Geometry: final body of the model. Coordinates: model frame, mm. A direction names the side the tool comes from. Give positions to 0.01 mm unless a question says otherwise; leave off trailing zeros. Loops run counter-clockwise (first coordinate to the right, second up) from the corner with the lowest first, then second, coordinate; pieces in that order, holes last. Notation, with made-up numbers: (-23.75, -22) -> (-18.75, -22) arc R13 ccw to (-18.75, 1) -> close; hole circle Ø2 at (-31.5, 45). An arc over 180 degrees is marked (long way). Answer in a Markdown table with one row per item. Add a question column.
1) Draft query along X for faces 1 (the flat face through (43, 43.18, -1)), 2 (the flat face through (4, 10.16, -60)), 3 (the flat face through (0, 21, -31)). Return one class per face: +X half, -X half, draft (parallel to the pull), parting line (faces both ways), or undercut.
2) Section query D-D (x = 5.08). Return the cut outline in (y, z).
3) Access query for faces 4 (the flat face through (60, 21, 0)), 5 (the flat face through (7.62, 8, -58)). Directions: +Z, -Z, +X, -X, +Y, -Y. A direction counts if a zero-diameter tool reaches every point of the face in a straight line with its end or side. Return the directions, or none.
4) First-contact query: P1, Ø0.8, axis at x = 5.5, z = -58.5, coming from the +Y side; P2, Ø3, axis at x = 99, z = -45, coming from the +Y side. Flat tips, straight axial feed; report the tip coordinate or a pass-through.
5) Section query C-C (x = 50.5). Return the cut outline in (y, z), plus the area to 3 significant figures.
6) Section query A-A (y = 22.5). Return the cut outline in (x, z).
7) Section query B-B (z = -58.42). Return the cut outline in (x, y).
8) Line query: line 1 (Z direction, x = 74.5, y = 38); line 2 (X direction, y = 8.5, z = -49); line 3 (Y direction, x = 5, z = -47). Output: solid intervals per line, ascending. Write a range as from..to.
```python
from build123d import *

# Parameters (mm, degrees)
SKETCH1_W           = 121.92
SKETCH1_H           = 63.5
BOSS_EXTRUDE1_DEPTH = 5.08
SKETCH2_W           = 121.92
SKETCH2_H           = 63.5
SKETCH2_W_2         = 116.84
SKETCH2_H_2         = 58.42
BOSS_EXTRUDE2_DEPTH = 38.1
SKETCH4_W           = 5.08
SKETCH4_H           = 5.08
BOSS_EXTRUDE3_DEPTH = 5.08
SKETCH5_R           = 1.27
BOSS_EXTRUDE4_DEPTH = 5.08


with BuildPart() as part:
    # Sketch1 → Boss-Extrude1 (new body)
    with BuildSketch(Plane(origin=(0, 0, 0), x_dir=(1, 0, 0), z_dir=(0, 1, 0))):
        with Locations((60.96, 31.75)):
            Rectangle(SKETCH1_W, SKETCH1_H)
    extrude(amount=BOSS_EXTRUDE1_DEPTH)

    # Sketch2 → Boss-Extrude2 (add)
    with BuildSketch(Plane(origin=(0, 5.08, 0), x_dir=(1, 0, 0), z_dir=(0, 1, 0))):
        with Locations((60.96, 31.75)):
            Rectangle(SKETCH2_W, SKETCH2_H)
        with Locations((60.96, 31.75)):
            Rectangle(SKETCH2_W_2, SKETCH2_H_2, mode=Mode.SUBTRACT)
    extrude(amount=BOSS_EXTRUDE2_DEPTH)

    # Sketch4 → Boss-Extrude3 (add)
    with BuildSketch(Plane(origin=(0, 5.08, 0), x_dir=(1, 0, 0), z_dir=(0, 1, 0))):
        with Locations((5.08, 58.42)):
            Rectangle(SKETCH4_W, SKETCH4_H)
        with Locations((116.84, 58.42)):
            Rectangle(SKETCH4_W, SKETCH4_H)
        with Locations((116.84, 5.08)):
            Rectangle(SKETCH4_W, SKETCH4_H)
        with Locations((5.08, 5.08)):
            Rectangle(SKETCH4_W, SKETCH4_H)
    extrude(amount=BOSS_EXTRUDE3_DEPTH)

    # Sketch5 → Boss-Extrude4 (add)
    with BuildSketch(Plane(origin=(0, 10.16, 0), x_dir=(1, 0, 0), z_dir=(0, 1, 0))):
        with Locations(Location((5.08, 58.42, 0), (0, 0, 270))):
            Circle(SKETCH5_R)
        with Locations(Location((116.84, 58.42, 0), (0, 0, 270))):
            Circle(SKETCH5_R)
        with Locations(Location((116.84, 5.08, 0), (0, 0, 270))):
            Circle(SKETCH5_R)
        with Locations(Location((5.08, 5.08, 0), (0, 0, 270))):
            Circle(SKETCH5_R)
    extrude(amount=BOSS_EXTRUDE4_DEPTH)


solid = part.part
```
Evaluation:
| question | item | result |
|---|---|---|
| 1 | face 1 | draft |
| 1 | face 2 | undercut |
| 1 | face 3 | -X half |
| 2 | outline | (0, -63.5) -> (43.18, -63.5) -> (43.18, -60.96) -> (10.16, -60.96) -> (10.16, -59.69) -> (15.24, -59.69) -> (15.24, -57.15) -> (10.16, -57.15) -> (10.16, -55.88) -> (5.08, -55.88) -> (5.08, -7.62) -> (10.16, -7.62) -> (10.16, -6.35) -> (15.24, -6.35) -> (15.24, -3.81) -> (10.16, -3.81) -> (10.16, -2.54) -> (43.18, -2.54) -> (43.18, 0) -> (0, 0) -> close |
| 3 | face 4 | +Z, +X, -X, +Y, -Y |
| 3 | face 5 | +Y |
| 4 | P1 | y = 15.24 |
| 4 | P2 | y = 5.08 |
| 5 | outline | (0, -63.5) -> (43.18, -63.5) -> (43.18, -60.96) -> (5.08, -60.96) -> (5.08, -2.54) -> (43.18, -2.54) -> (43.18, 0) -> (0, 0) -> close |
| 5 | area | 516 mm² |
| 6 | outline | (0, -63.5) -> (121.92, -63.5) -> (121.92, 0) -> (0, 0) -> close; hole (2.54, -60.96) -> (119.38, -60.96) -> (119.38, -2.54) -> (2.54, -2.54) -> close |
| 7 | outline | (0, 0) -> (121.92, 0) -> (121.92, 43.18) -> (119.38, 43.18) -> (119.38, 10.16) -> (118.11, 10.16) -> (118.11, 15.24) -> (115.57, 15.24) -> (115.57, 10.16) -> (114.3, 10.16) -> (114.3, 5.08) -> (7.62, 5.08) -> (7.62, 10.16) -> (6.35, 10.16) -> (6.35, 15.24) -> (3.81, 15.24) -> (3.81, 10.16) -> (2.54, 10.16) -> (2.54, 43.18) -> (0, 43.18) -> close |
| 8 | line 1 | -63.5..-60.96, -2.54..0 |
| 8 | line 2 | 0..2.54, 119.38..121.92 |
| 8 | line 3 | 0..5.08 |
